Build history of the part. All positions in model axes, mm. Face numbers are marked on the shaded views. A direction names the side the tool comes from. Round coordinates to 2 decimals unless told otherwise and drop trailing zeros. Order: outer loops, then holes, each group sorted by start corner. A loop starts at its lowest first (then second) coordinate and runs counter-clockwise, first axis right, second up. Notation, with made-up numbers: (68, 80) - (101, 80) arc R13 ccw to (101, 92) - close; hole circle Ø11 at (-37.5, 9.25). An arc over 180 degrees is marked (long way). One line per question, with ' | ' between items. Start each with the question number.
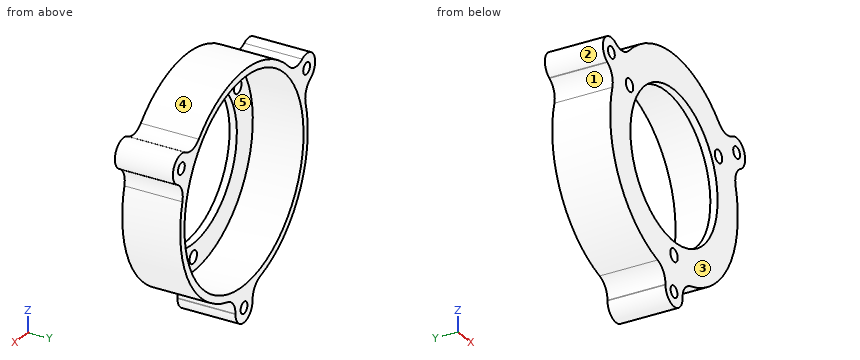
from build123d import *

# Parameters (mm, degrees)
SKETCH1_R           = 30
SKETCH1_R_2         = 20.5
BOSS_EXTRUDE1_DEPTH = 16
SKETCH2_R           = 28
CUT_EXTRUDE1_DEPTH  = 14
BOSS_EXTRUDE2_START = -16
SKETCH4_R           = 4
SKETCH4_R_2         = 1.6
BOSS_EXTRUDE2_DEPTH = 16
FILLET1_R           = 5
SKETCH5_R           = 1.75
CUT_EXTRUDE2_DEPTH  = 53.521985177


with BuildPart() as part:
    # Sketch1 → Boss-Extrude1 (new body)
    with BuildSketch(Plane(origin=(0, 0, 0), x_dir=(1, 0, 0), z_dir=(0, 1, 0))):
        with Locations(Location((0, 0, 0), (0, 0, 270))):
            Circle(SKETCH1_R)
        with Locations(Location((0, 0, 0), (0, 0, 270))):
            Circle(SKETCH1_R_2, mode=Mode.SUBTRACT)
    extrude(amount=BOSS_EXTRUDE1_DEPTH)

    # Sketch2 → Cut-Extrude1 (cut)
    with BuildSketch(Plane(origin=(0, 16, 0), x_dir=(1, 0, 0), z_dir=(0, 1, 0))):
        with Locations(Location((0, 0, 0), (0, 0, 270))):
            Circle(SKETCH2_R)
    extrude(amount=-CUT_EXTRUDE1_DEPTH, mode=Mode.SUBTRACT)

    # Sketch4 → Boss-Extrude2 (add)
    # profile 1 of 9: a face of its own
    with BuildSketch(Plane(origin=(0, 16, 0), x_dir=(1, 0, 0), z_dir=(0, 1, 0)).offset(BOSS_EXTRUDE2_START)):
        with Locations((-29.444863729, -17)):
            Circle(SKETCH4_R)
        with Locations(Location((-29.444863729, -17, 0), (0, 0, 270))):
            Circle(SKETCH4_R_2, mode=Mode.SUBTRACT)
    # profile 2 of 9: a face of its own
    with BuildSketch(Plane(origin=(0, 16, 0), x_dir=(1, 0, 0), z_dir=(0, 1, 0)).offset(BOSS_EXTRUDE2_START)):
        with BuildLine():
            ThreePointArc((-23.897530801, -18.135821504), (-24.988384694, -16.600621385), (-25.980762095, -15.000000032))
            ThreePointArc((-25.980762095, -15.000000032), (-25.581160419, -15.964723837), (-25.444863729, -17))
            ThreePointArc((-25.444863729, -17), (-25.92341304, -18.897204534), (-27.244556251, -20.340456107))
            Line((-27.244556251, -20.340456107), (-23.897530801, -18.135821504))
        make_face()
    # profile 3 of 9: a face of its own
    with BuildSketch(Plane(origin=(0, 16, 0), x_dir=(1, 0, 0), z_dir=(0, 1, 0)).offset(BOSS_EXTRUDE2_START)):
        with BuildLine():
            ThreePointArc((-25.980762095, -15.000000032), (-26.92494299, -13.230549686), (-27.748786379, -11.401967132))
            Line((-27.748786379, -11.401967132), (-31.444863729, -13.535898385))
            ThreePointArc((-31.444863729, -13.535898385), (-28.40958753, -13.1362967), (-25.980762095, -15.000000032))
        make_face()
    # profile 4 of 9: a face of its own
    with BuildSketch(Plane(origin=(0, 16, 0), x_dir=(1, 0, 0), z_dir=(0, 1, 0)).offset(BOSS_EXTRUDE2_START)):
        with Locations((0, 34)):
            Circle(SKETCH4_R)
        with Locations(Location((0, 34, 0), (0, 0, 270))):
            Circle(SKETCH4_R_2, mode=Mode.SUBTRACT)
    # profile 5 of 9: a face of its own
    with BuildSketch(Plane(origin=(0, 16, 0), x_dir=(1, 0, 0), z_dir=(0, 1, 0)).offset(BOSS_EXTRUDE2_START)):
        with BuildLine():
            Line((4, 29.732137495), (4, 34))
            ThreePointArc((4, 34), (2.828427119, 31.171572869), (-1.7e-08, 30))
            ThreePointArc((-1.7e-08, 30), (2.00447937, 29.932959467), (4, 29.732137495))
        make_face()
    # profile 6 of 9: a face of its own
    with BuildSketch(Plane(origin=(0, 16, 0), x_dir=(1, 0, 0), z_dir=(0, 1, 0)).offset(BOSS_EXTRUDE2_START)):
        with BuildLine():
            ThreePointArc((-1.7e-08, 30), (-2.828427131, 31.171572881), (-4, 34))
            Line((-4, 34), (-4, 29.732137495))
            ThreePointArc((-4, 29.732137495), (-2.004479388, 29.932959466), (-1.7e-08, 30))
        make_face()
    # profile 7 of 9: a face of its own
    with BuildSketch(Plane(origin=(0, 16, 0), x_dir=(1, 0, 0), z_dir=(0, 1, 0)).offset(BOSS_EXTRUDE2_START)):
        with BuildLine():
            ThreePointArc((27.244556251, -20.340456107), (25.552370926, -17.921140477), (25.980761986, -15.00000022))
            ThreePointArc((25.980761986, -15.00000022), (24.988384634, -16.600621476), (23.897530801, -18.135821504))
            Line((23.897530801, -18.135821504), (27.244556251, -20.340456107))
        make_face()
    # profile 8 of 9: a face of its own
    with BuildSketch(Plane(origin=(0, 16, 0), x_dir=(1, 0, 0), z_dir=(0, 1, 0)).offset(BOSS_EXTRUDE2_START)):
        with BuildLine():
            Line((31.237629839, -13.424249775), (27.74612946, -11.408431091))
            ThreePointArc((27.74612946, -11.408431091), (26.923401686, -13.233685868), (25.980761986, -15.00000022))
            ThreePointArc((25.980761986, -15.00000022), (28.296348137, -13.168432183), (31.237629839, -13.424249775))
        make_face()
    # profile 9 of 9: a face of its own
    with BuildSketch(Plane(origin=(0, 16, 0), x_dir=(1, 0, 0), z_dir=(0, 1, 0)).offset(BOSS_EXTRUDE2_START)):
        with Locations((29.444863729, -17)):
            Circle(SKETCH4_R)
        with Locations(Location((29.444863729, -17, 0), (0, 0, 270))):
            Circle(SKETCH4_R_2, mode=Mode.SUBTRACT)
    extrude(amount=BOSS_EXTRUDE2_DEPTH)

    # Fillet1
    fillet1_edges = [part.edges().sort_by_distance(p)[0] for p in [
        (23.897530801, 8, 18.135821504),
        (27.74612946, 8, 11.408431091),
        (4, 8, -29.732137495),
        (-4, 8, -29.732137495),
        (-27.748786379, 8, 11.401967132),
        (-23.897530801, 8, 18.135821504),
    ]]
    fillet(fillet1_edges, radius=FILLET1_R)

    # Sketch5 → Cut-Extrude2 (cut, through all)
    with BuildSketch(Plane(origin=(0, 2, 0), x_dir=(1, 0, 0), z_dir=(0, 1, 0))):
        with Locations(Location((0, 24.15056176, 0), (0, 0, 270))):
            Circle(SKETCH5_R)
        with Locations(Location((-20.915, -12.07528088, 0), (0, 0, 270))):
            Circle(SKETCH5_R)
        with Locations(Location((20.915, -12.07528088, 0), (0, 0, 270))):
            Circle(SKETCH5_R)
    extrude(amount=-CUT_EXTRUDE2_DEPTH, mode=Mode.SUBTRACT)


solid = part.part
Item 1: Slice it at C-C (x = -11). Write the cut outline in (y, z), plus the area to 3 significant figures.
Item 2: Pull direction Z, two halves, no side cores. Call the marked faces 1, 2 and 3: released by +Z, released by -Z, zero draft, split by the parting line, or undercut.
Item 3: Slice it at D-D (z = 17). Write the cut outline in (x, y), plus the area to 3 significant figures.
Item 4: Slice it at B-B (z = 4). Write the cut outline in (x, y).
Item 5: 3-axis set-ups, long thin cutter, end or side, ignore diameter. For the marked faces 4 and 5: which of +Z, -Z, +X, -X, +Y, -Y reach the whole face in a straight line?
Item 6: Slice it at A-A (x = 0). Write the cut outline in (y, z), plus the area to 3 significant figures.
Item 7: Wall check: line 1 along X through (y, z) = (8, 0); line 2 along X through (y, z) = (12.5, -33); line 3 along Z through (x, y) = (-19, 13.5). Give the ranges that are in metal, low to high. Write a range as [from, to].
Item 8: Pin check, flat tips, straight feed: pin 1 (1.9 mm diameter, centred on x = -29.44, z = 17, fed in from +Y); pin 2 (4 mm diameter, centred on x = 2.5, y = 4.5, fed in from +Z); pin 3 (1 mm diameter, centred on x = -24, z = -18.5, fed in from -Y); pin 4 (1.5 mm diameter, centred on x = 3.5, y = 7.5, fed in from -Z). Stop position of each tip, or through.
A:
1) outline: (0, -27.91) - (16, -27.91) - (16, -25.75) - (2, -25.75) - (2, -17.3) - (0, -17.3) - close; (0, 17.3) - (2, 17.3) - (2, 25.75) - (16, 25.75) - (16, 27.91) - (0, 27.91) - close | area: 103 mm^2
2) face 1: undercut | face 2: split by the parting line | face 3: zero draft
3) outline: (-33.44, 0) - (-31.04, 0) - (-31.04, 16) - (-33.44, 16) - close; (-27.84, 0) - (-11.46, 0) - (-11.46, 2) - (-22.25, 2) - (-22.25, 16) - (-27.84, 16) - close; (11.46, 0) - (27.84, 0) - (27.84, 16) - (22.25, 16) - (22.25, 2) - (11.46, 2) - close; (31.04, 0) - (33.44, 0) - (33.44, 16) - (31.04, 16) - close | area: 299 mm^2
4) outline: (-29.73, 0) - (-20.11, 0) - (-20.11, 2) - (-27.71, 2) - (-27.71, 16) - (-29.73, 16) - close; (20.11, 0) - (29.73, 0) - (29.73, 16) - (27.71, 16) - (27.71, 2) - (20.11, 2) - close
5) face 4: +Z, +Y, -Y | face 5: +Y
6) outline: (0, -38) - (16, -38) - (16, -35.6) - (0, -35.6) - close; (0, -32.4) - (16, -32.4) - (16, -28) - (2, -28) - (2, -25.9) - (0, -25.9) - close; (0, -22.4) - (2, -22.4) - (2, -20.5) - (0, -20.5) - close; (0, 20.5) - (2, 20.5) - (2, 28) - (16, 28) - (16, 30) - (0, 30) - close | area: 164 mm^2
7) line 1: [-30, -28], [28, 30] | line 2: [-4.07, -1.25], [1.25, 4.07] | line 3: [-23.22, -20.57], [20.57, 23.22]
8) pin 1: through | pin 2: z = 30 | pin 3: y = 0 | pin 4: z = -36.9
